Check sheet for the modelled part. Datum: model origin and axes. Units: mm. Face numbers are marked on the shaded views. A direction names the side the tool comes from. Give positions to 0.01 mm unless a question says otherwise; leave off trailing zeros. Write each loop counter-clockwise with the first axis right and the second up, starting at its lowest first coordinate (ties: lowest second). Pieces come first, ordered by that corner, then holes. Notation, with made-up numbers: M -5.75,46 L 5.25,46 A33 ccw 5.25,79 Z; hole C -30,9 d10. An arc over 180 degrees is marked long. Write each question's results on one line, items separated by ' | '. Start each with the question number.
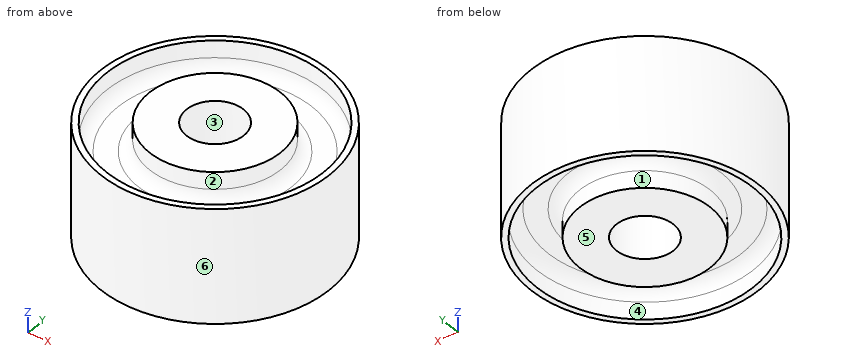
from build123d import *

# Parameters (mm, degrees)
BOSS_EXTRUDE1_DEPTH      = 25.4
BOSS_EXTRUDE1_DEPTH_BACK = 25.4
SKETCH1_R                = 50.8
SKETCH3_R                = 12.7
CUT_EXTRUDE2_DEPTH       = 88.988181024


with BuildPart() as part:
    # Sketch1 → Boss-Extrude1 (new, two sides: drawn at the far end of the back side and taken through both)
    with BuildSketch(Plane.XY.offset(-BOSS_EXTRUDE1_DEPTH_BACK)):
        Circle(SKETCH1_R)
    extrude(amount=BOSS_EXTRUDE1_DEPTH + BOSS_EXTRUDE1_DEPTH_BACK)

    # Sketch3 → Cut-Extrude2 (cut, through all)
    with BuildSketch(Plane.XY.offset(25.4)):
        Circle(SKETCH3_R)
    extrude(amount=-CUT_EXTRUDE2_DEPTH, mode=Mode.SUBTRACT)

    # Cut-Sweep1: sweep along a path in Sketch4
    with BuildLine(Plane.XY.offset(25.4)) as cut_sweep1_path:
        CenterArc((0, 0), 38.1, 0, 360)
    # Sketch7 → Cut-Sweep1 (sweep, cut)
    with BuildSketch(Plane(origin=(0, 0, 0), x_dir=(0, 0, -1), z_dir=(1, 0, 0))):
        with BuildLine():
            Line((-25.4, 48.177038495), (-17.78, 48.177038495))
            ThreePointArc((-17.78, 48.177038495), (-14.187897552, 46.689140943), (-12.7, 43.097038495))
            Line((-12.7, 43.097038495), (-12.7, 34.207038495))
            ThreePointArc((-12.7, 34.207038495), (-14.187897552, 30.614936046), (-17.78, 29.127038495))
            Line((-17.78, 29.127038495), (-25.4, 29.127038495))
            Line((-25.4, 29.127038495), (-25.4, 48.177038495))
        make_face()
    cut_sweep1 = sweep(path=cut_sweep1_path.line, mode=Mode.SUBTRACT)

    # Mirror1: Cut-Sweep1 across plane
    add(cut_sweep1.mirror(Plane.XY), mode=Mode.SUBTRACT)


solid = part.part
Q1. Section check A-A on z = -20. Record the boundary of the cut face in (x, y).
Q2. Release check for a two-part mould opening along X. For the marked faces 4, 5 and 6 record: pulls with the +X half, pulls with the -X half, needs draft (parallel to the pull), parting line crosses it, or undercut.
Q3. Depth check by flat-ended pin: pin 1 Ø15 at (x, y) = (0, 0) entering from +Z; pin 2 Ø1.5 at (x, y) = (-27.5, 38) entering from +Z; pin 3 Ø1.5 at (y, z) = (-16, 14.5) entering from +X; pin 4 Ø1.5 at (x, z) = (-6, 7.5) entering from -Y. Enter the tip coordinate at first touch or a pass-through.
Q4. Tool access check on the marked faces 1, 2 and 3. Record the directions out of +Z, -Z, +X, -X, +Y, -Y that give a thin tool (end or side, any length) a straight path to the whole face; none if there is none.
Q5. Scan lines: L1, parallel to Y at x = 0, z = -20; L2, parallel to Y at x = 0, z = -1; L3, parallel to Y at x = -24.5, z = -18.5. Record each from-to range of solid material in increasing order.
Q6. Section check B-B on z = 5.5. Record the boundary of the cut face in (x, y), plus the area to 3 significant figures.
Check result:
1) outline: C 0,0 d101.6; C 0,0 d58.25; hole C 0,0 d96.35; hole C 0,0 d25.4
2) face 4: undercut | face 5: needs draft | face 6: parting line crosses it
3) pin 1: through | pin 2: z = 15.54 | pin 3: x = 48.46 | pin 4: y = -50.53
4) face 1: -Z | face 2: +Z | face 3: +Z, -Z
5) L1: -50.8 to -48.18, -29.13 to -12.7, 12.7 to 29.13, 48.18 to 50.8 | L2: -50.8 to -12.7, 12.7 to 50.8 | L3: -44.5 to -41.48, -15.75 to 15.75, 41.48 to 44.5
6) outline: C 0,0 d101.6; hole C 0,0 d25.4 | area: 7,600 mm^2
